from build123d import *

# Parameters (mm, degrees)
BOSS_EXTRUDE1_DEPTH = 5.08
SKETCH2_W           = 34.036
SKETCH2_H           = 12.7
BOSS_EXTRUDE2_DEPTH = 5.08


with BuildPart() as part:
    # Sketch1 → Boss-Extrude1 (new body)
    with BuildSketch(Plane.XY):
        with BuildLine():
            ThreePointArc((4.89576896, 33.263952472), (25.4, 16.631976236), (45.90423104, 33.263952472))
            Line((45.90423104, 33.263952472), (50.8, 33.263952472))
            Line((50.8, 33.263952472), (50.8, 0))
            Line((50.8, 0), (0, 0))
            Line((0, 0), (0, 33.263952472))
            Line((0, 33.263952472), (4.89576896, 33.263952472))
        make_face()
    extrude(amount=BOSS_EXTRUDE1_DEPTH)

    # Sketch2 → Boss-Extrude2 (add)
    with BuildSketch(Plane(origin=(0, 0, 0), x_dir=(0, 0, -1), z_dir=(1, 0, 0))):
        with Locations((-22.098, 6.35)):
            Rectangle(SKETCH2_W, SKETCH2_H)
    extrude(amount=BOSS_EXTRUDE2_DEPTH)


solid = part.part
Model file for the job. Use its own axes, mm. A direction names the side the tool comes from. Round coordinates to 2 decimals unless told otherwise and drop trailing zeros. Order: outer loops, then holes, each group sorted by start corner. A loop starts at its lowest first (then second) coordinate and runs counter-clockwise, first axis right, second up.
(1) Drill centre lines: line 1 (X direction, y = 4, z = 6.5); line 2 (X direction, y = 29.5, z = 3). Where is each one in solid material? Low to high.
(2) Band-saw the part on B-B (z = 25). List the corners of the cut face in (x, y), then the cut area to 3 significant figures.
(3) 3-axis set-ups, long thin cutter, end or side, ignore diameter. For faces 5 (the face through (5.08, 6, 22)), 6 (the face through (16, 0, 4)), 7 (the face through (3, 12.7, 22)): which of +Z, -Z, +X, -X, +Y, -Y reach the whole face in a straight line?
(4) Pin check, flat tips, straight feed: pin 1 (6 mm diameter, centred on y = 3.5, z = 21.5, fed in from +X); pin 2 (12 mm diameter, centred on x = 12.5, y = 12.5, fed in from +Z); pin 3 (1.5 mm diameter, centred on x = 2.5, z = 21, fed in from +Y). Stop position of each tip, or through.
(5) Band-saw the part on C-C (y = 3.5). List the corners of the cut face in (x, z), then the cut area to 3 significant figures.
(6) Band-saw the part on D-D (x = 6). List the corners of the cut face in (y, z).
(7) Pull direction X, two halves, no side cores. Call faces 1 (the face through (25, 16.636, 2.504)), 2 (the face through (0, 9, 15)), 3 (the face through (2, 33.264, 3)), 4 (the face through (50.8, 17, 3)): released by +X, released by -X, zero draft, split by the parting line, or undercut.
(8) Band-saw the part on A-A (y = 31). List the corners of the cut face in (x, z).
Verdict:
1. line 1: x = 0 to 5.08
1. line 2: x = 0 to 6.07, 44.73 to 50.8
2. outline: (0, 0) - (5.08, 0) - (5.08, 12.7) - (0, 12.7) - close
2. area: 64.5 mm2
3. face 5: +Z, +X, +Y, -Y
3. face 6: +Z, -Z, +X, -X, -Y
3. face 7: +Z, +X, -X, +Y
4. pin 1: stops at x = 5.08
4. pin 2: stops at z = 5.08
4. pin 3: stops at y = 12.7
5. outline: (0, 0) - (50.8, 0) - (50.8, 5.08) - (5.08, 5.08) - (5.08, 39.12) - (0, 39.12) - close
5. area: 431 mm2
6. outline: (0, 0) - (29.67, 0) - (29.67, 5.08) - (0, 5.08) - close
7. face 1: undercut
7. face 2: released by -X
7. face 3: zero draft
7. face 4: released by +X
8. outline: (0, 0) - (5.51, 0) - (5.51, 5.08) - (0, 5.08) - close; (45.29, 0) - (50.8, 0) - (50.8, 5.08) - (45.29, 5.08) - close
